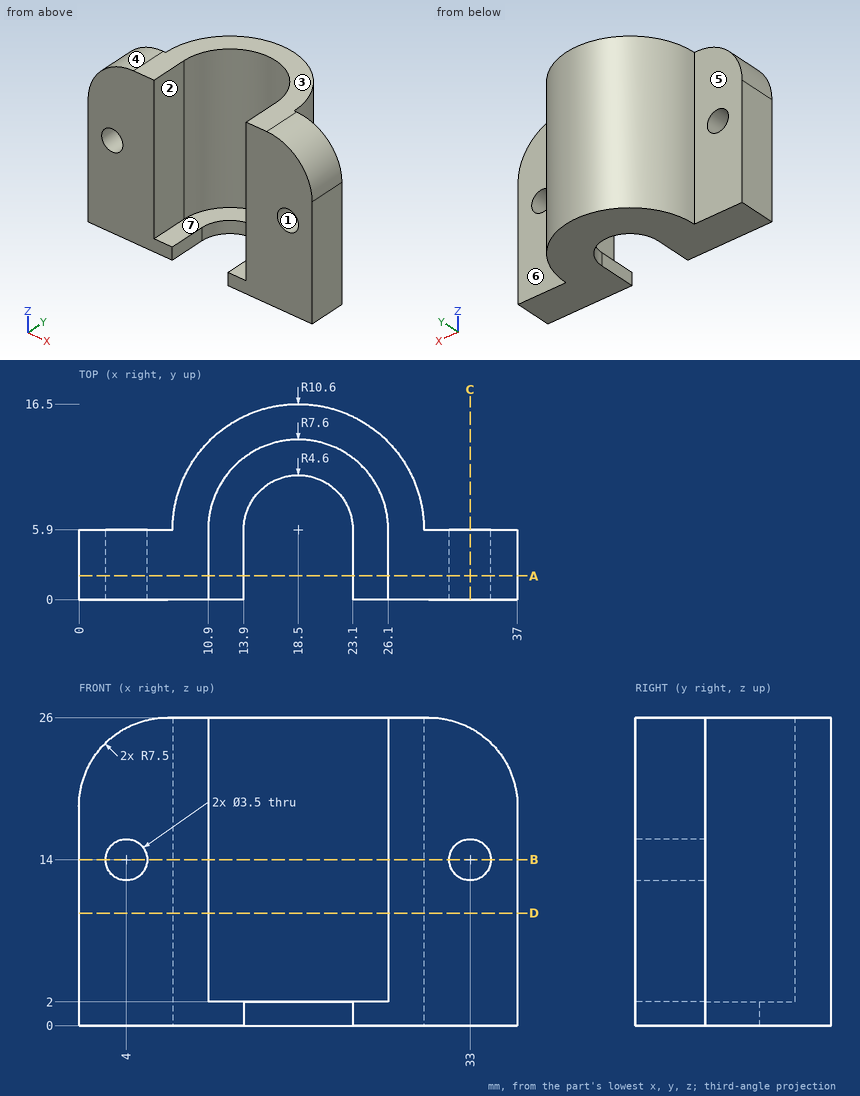
Check sheet for the drawn part. Datum: minimum x, y, z corner. Units: mm. A direction names the side the tool comes from. Give positions to 0.01 mm unless a question says otherwise; leave off trailing zeros. Write each loop counter-clockwise with the first axis right and the second up, starting at its lowest first coordinate (ties: lowest second). Pieces come first, ordered by that corner, then holes. Notation, with made-up numbers: M 28,-34 L 77,-34 A28 ccw 77,-3 Z; hole C -33,-12 d4. An arc over 180 degrees is marked long. Write item = value, one per line.
(1) Sectioned sample at D-D (z = 9.5). Record the cut outline in (x, y).
Found:
outline = M 0,0 L 10.9,0 L 10.9,5.9 A7.6 cw 26.1,5.9 L 26.1,0 L 37,0 L 37,5.9 L 29.1,5.9 A10.6 ccw 7.9,5.9 L 0,5.9 Z
(2) Access from +Z, -Z, +X, -X, +Y, -Y to the whole of each face (thin tool, end or side, straight path). Record for the marked faces 5, 6 and 7.
Found:
face_5 = +Z, -Z, -X, +Y
face_6 = +Z, -Z, +X, +Y
face_7 = +Z, -Y
(3) Material ranges on line 1 (X direction, y = 4.65, z = 14); line 2 (X direction, y = 1.25, z = 8); line 3 (Z direction, x = 25, y = 7), recorded low to high.
Found:
line_1 = 0 to 2.25, 5.75 to 10.9, 26.1 to 31.25, 34.75 to 37
line_2 = 0 to 10.9, 26.1 to 37
line_3 = 0 to 2
(4) Sectioned sample at C-C (x = 33). Record the cut outline in (y, z), then the cut area to 3 significant figures.
Found:
outline = M 0,0 L 5.9,0 L 5.9,12.25 L 0,12.25 Z; M 0,15.75 L 5.9,15.75 L 5.9,25.13 L 0,25.13 Z
area = 128 mm2
(5) Go/stop test with flat-tipped pins: pin 1 Ø8 at (y, z) = (14.5, 6.5) entering from -X; pin 2 Ø1 at (x, z) = (15.5, 13.5) entering from -Y; pin 3 Ø8.5 at (x, z) = (34.5, 16.5) entering from +Y. Record where each tip stops, or that it passes through.
Found:
pin_1 = 8.95
pin_2 = 12.65
pin_3 = 5.9
(6) Sectioned sample at B-B (z = 14). Record the cut outline in (x, y).
Found:
outline = M 0,0 L 2.25,0 L 2.25,5.9 L 0,5.9 Z; M 5.75,0 L 10.9,0 L 10.9,5.9 A7.6 cw 26.1,5.9 L 26.1,0 L 31.25,0 L 31.25,5.9 L 29.1,5.9 A10.6 ccw 7.9,5.9 L 5.75,5.9 Z; M 34.75,0 L 37,0 L 37,5.9 L 34.75,5.9 Z
(7) Draft check along X on the marked faces 1, 2, 3 and 4. Enter one of: released by +X, released by -X, zero draft, split by the parting line, or undercut.
Found:
face_1 = undercut
face_2 = undercut
face_3 = zero draft
face_4 = released by -X
(8) Sectioned sample at A-A (y = 2). Record the cut outline in (x, z), then the cut area to 3 significant figures.
Found:
outline = M 0,0 L 13.9,0 L 13.9,2 L 10.9,2 L 10.9,26 L 7.5,26 A7.5 ccw 0,18.5 Z; M 23.1,0 L 37,0 L 37,18.5 A7.5 ccw 29.5,26 L 26.1,26 L 26.1,2 L 23.1,2 Z; hole C 4,14 d3.5; hole C 33,14 d3.5
area = 535 mm2
